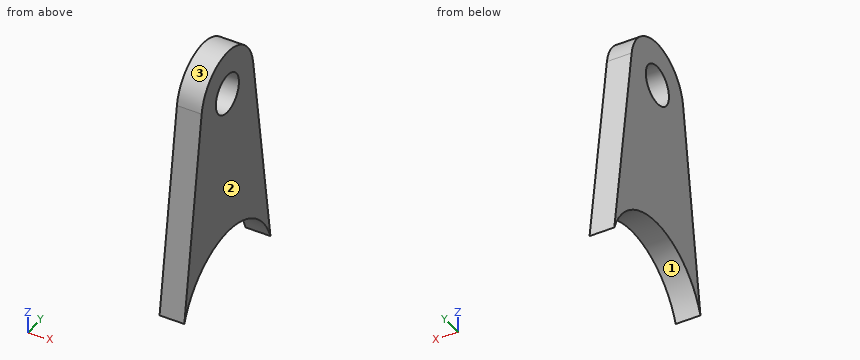
from build123d import *

# Parameters (mm, degrees)
BOSS_EXTRUDE1_DEPTH = 2.5


with BuildPart() as part:
    # Sketch1 → Boss-Extrude1 (new, symmetric)
    with BuildSketch(Plane.YZ):
        with BuildLine():
            ThreePointArc((-14.917620355, 5.429569775), (-9.105525927, 13.004038703), (0, 15.875))
            ThreePointArc((0, 15.875), (9.105525927, 13.004038703), (14.917620355, 5.429569775))
            Line((14.917620355, 5.429569775), (8.908095127, 47.157903431))
            ThreePointArc((8.908095127, 47.157903431), (0, 54.875), (-8.908095127, 47.157903431))
            Line((-8.908095127, 47.157903431), (-14.917620355, 5.429569775))
        make_face()
        with BuildLine():
            ThreePointArc((4, 45.875), (2.828427125, 43.046572875), (0, 41.875))
            ThreePointArc((0, 41.875), (-2.828427125, 48.703427125), (4, 45.875))
        make_face(mode=Mode.SUBTRACT)
    extrude(amount=BOSS_EXTRUDE1_DEPTH, both=True)


solid = part.part
Geometry check sheet. Reference: the model listing, model coordinates, mm. Face numbers are marked on the shaded views. Coordinates: 2 decimals unless noted, no trailing zeros. Order: outer loops, then holes, each group sorted by start corner. A loop starts at its lowest first (then second) coordinate and runs counter-clockwise, first axis right, second up. Notation, with made-up numbers: (46, -27) -> (97, -27) arc R22 ccw to (97, 0) -> close; hole circle Ø9 at (60, 16). An arc over 180 degrees is marked (long way). Use a Markdown table: item, result. Add a question column.
1. Cross-section at D-D (z = 37). Enter the section's corners in (x, y), and give its area (3 significant figures).
2. Mould release check, pull along Y, two halves, no side actions. Record for the marked faces 1, 2 and 3: pulls with the +Y half, pulls with the -Y half, needs draft (parallel to the pull), parting line crosses it, or undercut.
3. Cross-section at B-B (z = 14). Enter the section's corners in (x, y).
4. Material ranges on L1, parallel to Z at x = 0.75, y = -0.25; L2, parallel to Y at x = -1.3, z = 11.5; L3, parallel to Y at x = -0.65, z = 12, recorded low to high.
5. Go/stop test with flat-tipped pins: pin 1 Ø7 at (y, z) = (0, 45.875) entering from -X; pin 2 Ø1.5 at (x, z) = (1.5, 33) entering from +Y; pin 3 Ø3 at (x, y) = (-1, 1) entering from -Z. Record where each tip stops, or that it passes through.
6. Cross-section at A-A (y = 0). Enter the section's corners in (x, z) (3 decimals), and give its area (3 significant figures).
7. Cross-section at C-C (x = 0.1). Enter the section's corners in (y, z) (3 decimals).
Filled sheet:
| question | item | result |
|---|---|---|
| 1 | outline | (-2.5, -10.37) -> (2.5, -10.37) -> (2.5, 10.37) -> (-2.5, 10.37) -> close |
| 1 | area | 104 mm2 |
| 2 | face 1 | undercut |
| 2 | face 2 | needs draft |
| 2 | face 3 | parting line crosses it |
| 3 | outline | (-2.5, -13.68) -> (2.5, -13.68) -> (2.5, -7.48) -> (-2.5, -7.48) -> close; (-2.5, 7.48) -> (2.5, 7.48) -> (2.5, 13.68) -> (-2.5, 13.68) -> close |
| 4 | L1 | 15.87 to 41.88, 49.87 to 54.87 |
| 4 | L2 | -14.04 to -10.94, 10.94 to 14.04 |
| 4 | L3 | -13.97 to -10.39, 10.39 to 13.97 |
| 5 | pin 1 | through |
| 5 | pin 2 | y = 11.06 |
| 5 | pin 3 | z = 15.68 |
| 6 | outline | (-2.5, 15.875) -> (2.5, 15.875) -> (2.5, 41.875) -> (-2.5, 41.875) -> close; (-2.5, 49.875) -> (2.5, 49.875) -> (2.5, 54.875) -> (-2.5, 54.875) -> close |
| 6 | area | 155 mm2 |
| 7 | outline | (-14.918, 5.43) arc R15.875 cw to (14.918, 5.43) -> (8.908, 47.158) arc R9 ccw to (-8.908, 47.158) -> close; hole circle Ø8 at (0, 45.875) |
